The model under review builds one solid part; all positions refer to its coordinate system, in mm. Coordinates: 2 decimals unless noted, no trailing zeros. Loops run counter-clockwise (first coordinate to the right, second up) from the corner with the lowest first, then second, coordinate; pieces in that order, holes last. Notation, with made-up numbers: (-28, -34.75) - (-3, -34.75) arc R27 ccw to (-3, 3.25) - close; hole circle Ø7 at (-30.75, 36). An arc over 180 degrees is marked (long way). Use a Markdown table: item, result. Add a question column.
1) Add section B-B, the plane y = -31.5. Give the boundary of the cut face in (x, z).
2) Clearance check with flat-ended pins moving along their axes: pin 1 (1 mm diameter, centred on y = 81, z = 10, fed in from +X); pin 2 (3 mm diameter, centred on y = -60, z = -9.5, fed in from -X); pin 3 (6.5 mm diameter, centred on x = 0, y = 71, fed in from +Z). State where each tip first meets the part, or that it passes through.
3) Add section A-A, the plane x = 0. Give the boundary of the cut face in (y, z), and give its area (3 significant figures).
4) To check wall thickness, follow L1, parallel to X at y = 29.5, z = -0.5; L2, parallel to X at y = 97.5, z = 9.5; L3, parallel to X at y = 86.5, z = 10.25. State the ranges of each line that lie inside material, in increasing order. Write a range as [from, to].
5) Add section C-C, the plane y = 86. Give the boundary of the cut face in (x, z).
```python
from build123d import *

# Parameters (mm, degrees)
F0_R     = 12.5
F1_DEPTH = 150
F4_DEPTH = 4
F5_SIZE  = 1


with BuildPart() as f1:
    # F0 (on Front) → F1 (new body, symmetric)
    with BuildSketch(Plane.XZ):
        Circle(F0_R)
    extrude(amount=F1_DEPTH, both=True)

    # F3 (on offset) → F4 (cut)
    with BuildSketch(Plane.XY.offset(12.5)):
        with BuildLine():
            Line((4, 50), (4, 100))
            ThreePointArc((4, 100), (0, 104), (-4, 100))
            Line((-4, 100), (-4, 50))
            ThreePointArc((-4, 50), (0, 46), (4, 50))
        make_face()
    extrude(amount=-F4_DEPTH, mode=Mode.SUBTRACT)

    # F5
    f5_edges = [f1.edges().sort_by_distance(p)[0] for p in [
        (-12.5, 150, 0),
        (-12.5, -150, 0),
    ]]
    chamfer(f5_edges, length=F5_SIZE)


solid = f1.part
```
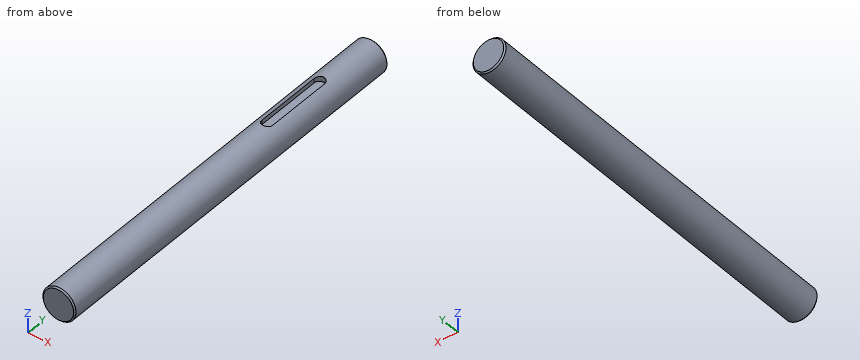
From the geometry:
| question | item | result |
|---|---|---|
| 1 | outline | circle Ø25 at (0, 0) |
| 2 | pin 1 | stops at x = 8.12 |
| 2 | pin 2 | stops at x = -9.6 |
| 2 | pin 3 | stops at z = 8.5 |
| 3 | outline | (-150, -11.5) - (-149, -12.5) - (149, -12.5) - (150, -11.5) - (150, 11.5) - (149, 12.5) - (104, 12.5) - (104, 8.5) - (46, 8.5) - (46, 12.5) - (-149, 12.5) - (-150, 11.5) - close |
| 3 | area | 7,270 mm^2 |
| 4 | L1 | x = [-12.49, 12.49] |
| 4 | L2 | x = [-8.12, -4], [4, 8.12] |
| 4 | L3 | x = [-7.15, -4], [4, 7.15] |
| 5 | outline | (-4, 8.5) - (-4, 11.84) arc R12.5 ccw (long way) to (4, 11.84) - (4, 8.5) - close |
